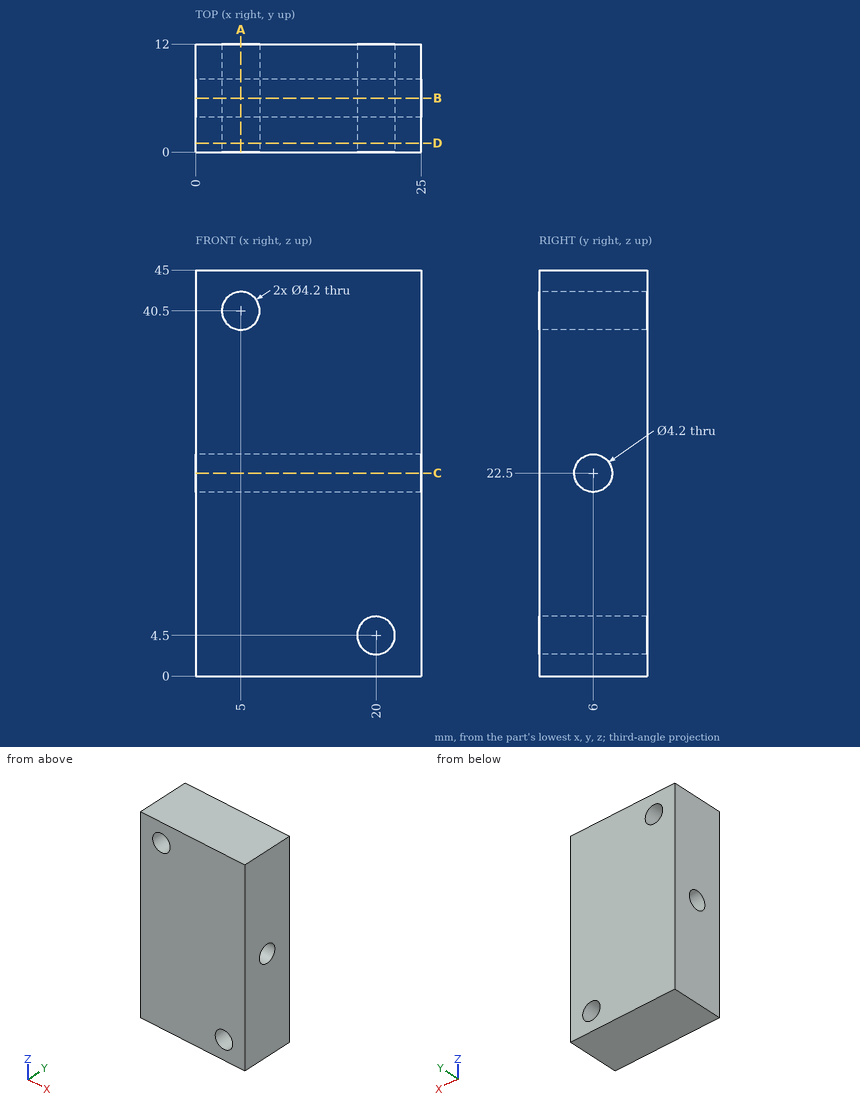
Verification items for this drawing (mm, ordinates from the low corner). Give positions to 0.01 mm unless a question says otherwise; leave off trailing zeros. Loops run counter-clockwise (first coordinate to the right, second up) from the corner with the lowest first, then second, coordinate; pieces in that order, holes last. Notation, with made-up numbers: M 53.25,-1.5 L 62.25,-1.5 A20 ccw 62.25,14.5 Z; hole C 37,53 d5. An arc over 180 degrees is marked long. Return JSON: item names as keys, results as strings. Group by question number.
1. Cross-section at B-B on y = 6. Record the boundary of the cut face in (x, z).
2. Cross-section at C-C on z = 22.5. Record the boundary of the cut face in (x, y), plus the area to 3 significant figures.
3. Cross-section at A-A on x = 5. Record the boundary of the cut face in (y, z), plus the area to 3 significant figures.
4. Go/stop test with a flat-tipped pin: pin 1 (3.5 mm diameter, centred on x = 20, z = 4.5, fed in from +Y). Record where the tip stops, or that it passes through.
5. Thickness scan on L1, parallel to Z at x = 5, y = 5; L2, parallel to X at y = 3.5, z = 40.5; L3, parallel to Z at x = 5, y = 3.5. Record the ranges inside material, lowest first.
6. Cross-section at D-D on y = 1. Record the boundary of the cut face in (x, z), plus the area to 3 significant figures.
Return value:
{
 "1": {"outline": "M 0,0 L 25,0 L 25,20.4 L 0,20.4 Z; M 0,24.6 L 25,24.6 L 25,45 L 0,45 Z; hole C 5,40.5 d4.2; hole C 20,4.5 d4.2"},
 "2": {"outline": "M 0,0 L 25,0 L 25,3.9 L 0,3.9 Z; M 0,8.1 L 25,8.1 L 25,12 L 0,12 Z", "area": "195 mm^2"},
 "3": {"outline": "M 0,0 L 12,0 L 12,38.4 L 0,38.4 Z; M 0,42.6 L 12,42.6 L 12,45 L 0,45 Z; hole C 6,22.5 d4.2", "area": "476 mm^2"},
 "4": {"pin 1": "through"},
 "5": {"L1": "0 to 20.65, 24.35 to 38.4, 42.6 to 45", "L2": "0 to 2.9, 7.1 to 25", "L3": "0 to 38.4, 42.6 to 45"},
 "6": {"outline": "M 0,0 L 25,0 L 25,45 L 0,45 Z; hole C 5,40.5 d4.2; hole C 20,4.5 d4.2", "area": "1,100 mm^2"}
}
